Autodesk Inventor part; units mm, degrees
ref_plane "YZ Plane" through (0, 0, 0) normal (1, 0, 0) x (0, 1, 0)
ref_plane "XZ Plane" through (0, 0, 0) normal (0, 1, 0) x (-1, 0, 0)
ref_plane "XY Plane" through (0, 0, 0) normal (0, 0, 1) x (1, 0, 0)
sketch "Sketch1" plane through (0, 0, 0) normal (1, 0, 0) x (0, 1, 0)
  line L0 (-12.5, 11) -> (12.5, 11)
  line L1 (12.5, 11) -> (12.5, -11)
  line L2 (12.5, -11) -> (-12.5, -11)
  line L3 (-12.5, -11) -> (-12.5, 11)
  line L4 (-12.5, 11) -> (12.5, -11) construction
  line L5 (12.5, 11) -> (-12.5, -11) construction
  line L6 (-9.5, 8) -> (9.5, 8)
  line L7 (9.5, 8) -> (9.5, -8)
  line L8 (9.5, -8) -> (-9.5, -8)
  line L9 (-9.5, -8) -> (-9.5, 8)
  line L10 (-9.5, 8) -> (9.5, -8) construction
  line L11 (9.5, 8) -> (-9.5, -8) construction
  line L12 (-9.5, 8) -> (-12.5, 8)
  line L13 (-12.5, 8) -> (-12.5, -8)
  line L14 (-12.5, -8) -> (-9.5, -8)
  line L15 (-9.5, -8) -> (-9.5, 8)
  line L16 (12.5, -11) -> (9.5, -11)
  line L17 (9.5, -11) -> (9.5, -21)
  line L18 (9.5, -21) -> (12.5, -21)
  line L19 (12.5, -21) -> (12.5, -11)
  point P0 (0, 0)
  point P1 (-12.5, 8)
  point P2 (9.5, -11)
  dimension "d0" = 25
  dimension "d1" = 22
  dimension "d2" = 19
  dimension "d3" = 16
  dimension "d4" = 3
  dimension "d5" = 10
extrude "Extrusion1" add sketch "Sketch1" along normal blind 10 contours L0 L1 L2 L3 L14 L8 L7 L6 L12 | L19 L18 L17 L2
sketch "Sketch2" plane through (0, 9.5, -8) normal (0, -1, 0) x (1, 0, 0)
  line L0 (10, 19) -> (10, 16)
  line L1 (0, 0) -> (0, -3)
  line L2 (10, 16) -> (0, 16)
  line L3 (0, 16) -> (0, 0)
  line L4 (0, 0) -> (10, 0)
  line L5 (10, 0) -> (10, 16)
  line L6 (5, 16) -> (5, 14)
  line L7 (5, 0) -> (5, 2)
  line L8 (5, 14) -> (5, 2) construction
  line L9 (3.35, 14) -> (3.35, 2)
  line L10 (6.65, 2) -> (6.65, 14)
  arc A0 (6.65, 14) -> (3.35, 14) centre (5, 14) ccw
  arc A1 (3.35, 2) -> (6.65, 2) centre (5, 2) ccw
  line L11 (0, -3) -> (0, -13)
  line L12 (10, -13) -> (0, -13)
  line L13 (0, -13) -> (0, -3)
  line L14 (0, -3) -> (10, -3)
  line L15 (10, -3) -> (10, -13)
  line L16 (5, -3) -> (5, -5)
  line L17 (5, -13) -> (5, -10)
  line L18 (5, -5) -> (5, -10) construction
  line L19 (3.35, -5) -> (3.35, -10)
  line L20 (6.65, -10) -> (6.65, -5)
  arc A2 (6.65, -5) -> (3.35, -5) centre (5, -5) ccw
  arc A3 (3.35, -10) -> (6.65, -10) centre (5, -10) ccw
  point P0 (0, 8)
  point P1 (5, 8)
  point P2 (5, -7.5)
  dimension "d8" = 2
  dimension "d9" = 2
  dimension "d10" = 3.3
  dimension "d11" = 2
  dimension "d12" = 3
  dimension "d13" = 3.3
extrude "Extrusion2" cut sketch "Sketch2" against normal through all contours A1 L9 A0 L10 | A2 L20 A3 L19
sketch "Sketch3" plane through (0, -12.5, 11) normal (0, 0, 1) x (1, 0, 0)
  line L0 (0, 0) -> (10, 0)
  line L1 (0, 22) -> (10, 22)
  line L2 (0, 0) -> (10, 0)
  line L3 (10, 0) -> (10, 22)
  line L4 (10, 22) -> (0, 22)
  line L5 (0, 22) -> (0, 0)
  line L6 (5, 22) -> (5, 18)
  line L7 (5, 0) -> (5, 4)
  line L8 (5, 18) -> (5, 4) construction
  line L9 (3.35, 18) -> (3.35, 4)
  line L10 (6.65, 4) -> (6.65, 18)
  arc A0 (6.65, 18) -> (3.35, 18) centre (5, 18) ccw
  arc A1 (3.35, 4) -> (6.65, 4) centre (5, 4) ccw
  point P0 (0, 12.5)
  point P1 (5, 11)
  dimension "d16" = 4
  dimension "d17" = 4
  dimension "d18" = 3.3
extrude "Extrusion3" cut sketch "Sketch3" against normal through all contours A1 L9 A0 L10
properties part number "BeltMount1"
For this review, take the finished solid that the model builds, in its own axes (mm). A direction names the side the tool comes from. Coordinates: 2 decimals unless noted, no trailing zeros. Order: outer loops, then holes, each group sorted by start corner. A loop starts at its lowest first (then second) coordinate and runs counter-clockwise, first axis right, second up. Notation, with made-up numbers: (-12.5, 63.25) -> (35.5, 63.25) arc R12 ccw to (35.5, 85.25) -> close; hole circle Ø8 at (-39.75, 13.5). An arc over 180 degrees is marked (long way). Return JSON: item names as keys, results as strings.
1. For line 1 (Z direction, x = 8.75, y = 3.5); line 2 (Z direction, x = 4.25, y = 11.5); line 3 (Y direction, x = 7.25, z = -3), list the stretches that pass through material, from the lowest coordinate up. Write a range as from..to.
Answer block:
{"line 1": "-11..-8, 8..11", "line 2": "-21..-19.47, -11.53..-7.47, 7.47..11", "line 3": "9.5..12.5"}
2. We need section D-D on y = 1. Write out the cut boundary in (x, z), and give its area (3 significant figures).
Answer block:
{"outline": "(0, -11) -> (3.35, -11) -> (3.35, -8) -> (0, -8) -> close; (0, 8) -> (3.35, 8) -> (3.35, 11) -> (0, 11) -> close; (6.65, -11) -> (10, -11) -> (10, -8) -> (6.65, -8) -> close; (6.65, 8) -> (10, 8) -> (10, 11) -> (6.65, 11) -> close", "area": "40.2 mm²"}
3. We need section C-C on y = -10.75. Write out the cut boundary in (x, z), and give its area (3 significant figures).
Answer block:
{"outline": "(0, -11) -> (10, -11) -> (10, -8) -> (0, -8) -> close; (0, 8) -> (10, 8) -> (10, 11) -> (0, 11) -> close", "area": "60.0 mm²"}
4. We need section A-A on z = -14. Write out the cut boundary in (x, y), and give its area (3 significant figures).
Answer block:
{"outline": "(0, 9.5) -> (3.35, 9.5) -> (3.35, 12.5) -> (0, 12.5) -> close; (6.65, 9.5) -> (10, 9.5) -> (10, 12.5) -> (6.65, 12.5) -> close", "area": "20.1 mm²"}
5. We need section B-B on x = 5. Write out the cut boundary in (y, z), and give its area (3 significant figures).
Answer block:
{"outline": "(-12.5, -11) -> (-10.15, -11) -> (-10.15, -8) -> (-12.5, -8) -> close; (-12.5, 8) -> (-10.15, 8) -> (-10.15, 11) -> (-12.5, 11) -> close; (7.15, -11) -> (9.5, -11) -> (9.5, -11.35) -> (12.5, -11.35) -> (12.5, -7.65) -> (9.5, -7.65) -> (9.5, -8) -> (7.15, -8) -> close; (7.15, 8) -> (9.5, 8) -> (9.5, 7.65) -> (12.5, 7.65) -> (12.5, 11) -> (7.15, 11) -> close; (9.5, -21) -> (12.5, -21) -> (12.5, -19.65) -> (9.5, -19.65) -> close", "area": "53.4 mm²"}
6. Machinability: for faces 4 (the cylindrical face through (4.96, 10.98, -7.65)), 5 (the flat face through (6.65, -2, 10)), 6 (the flat face through (3, -2, -8)), 7 (the flat face through (3, 9.5, -16)), which of the approach directions +Z, -Z, +X, -X, +Y, -Y give a long, thin tool a straight path to every point of the face, cutting with its end or side? Answer none if there is none.
Answer block:
{"face 4": "+Y, -Y", "face 5": "+Z, -Z", "face 6": "+X, -X, -Y", "face 7": "-Z, +X, -X, -Y"}
7. For pin 1 Ø1 at (x, y) = (2, -2.5) entering from -Z; pin 2 Ø3 at (x, z) = (3, -15.5) entering from -Y, all flat-tipped, find the tip position at first contact; note any pin that passes through.
Answer block:
{"pin 1": "z = -11", "pin 2": "y = 9.5"}
8. The part is to be moulded in two halves that separate along Z. For faces 1 (the flat face through (3, -1, -11)), 2 (the flat face through (10, 2.7, -8.5)), 3 (the cylindrical face through (5.04, 10.98, 7.65)), say which applies: +Z half, -Z half, draft (parallel to the pull), parting line (faces both ways), or undercut.
Answer block:
{"face 1": "-Z half", "face 2": "draft", "face 3": "undercut"}
